Can you work these out from the model? Positions are in its coordinate system, mm. A direction names the side the tool comes from. Round coordinates to 2 decimals unless told otherwise and drop trailing zeros. Write each loop counter-clockwise with the first axis right and the second up, starting at its lowest first coordinate (ties: lowest second). Pieces come first, ordered by that corner, then holes. Notation, with made-up numbers: (87.5, -24) -> (135.5, -24) arc R27 ccw to (135.5, 10) -> close; hole circle Ø6 at (53, 23). An arc over 180 degrees is marked (long way). Write item = value, one per line. Start each with the question number.
1) Imagine slicing it at B-B, the plane y = -6.25. Please give me the cut outline in (x, z).
2) For faces 4 (the face through (-3.55, -11, 2)), 5 (the face through (-7, -1, -9)), 6 (the face through (-8, -11, -13.8)), which set-ups out of +Z, -Z, +X, -X, +Y, -Y let a thin tool reach every point of the face, with its end or its side?
3) If I drill on line 1 (Z direction, x = 0, y = -7); line 2 (Z direction, x = 7, y = -6); line 3 (Y direction, x = 0, z = 2.5), over which ranges is the centre line in solid material (lowest first)?
4) Imagine slicing it at C-C, the plane x = 6. Please give me the cut outline in (y, z), then the cut area to 3 significant figures.
5) Imagine slicing it at D-D, the plane z = 3.75. Please give me the cut outline in (x, y), then the cut area to 3 significant figures.
6) Thinking about a two-plate mould opening in Y: for faces 1 (the face through (-7.35, -4.8, -12.56)), 2 (the face through (8.91, 0.27, -0.07)), 3 (the face through (8.2, -13, -9.7)), which applies, +Y half, -Y half, draft (parallel to the pull), parting line (faces both ways), or undercut?
7) Imagine slicing it at A-A, the plane y = -2.5. Please give me the cut outline in (x, z).
8) I'm going to push flat-ended pins straight in: pin 1 (1.7 mm diameter, centred on x = 6, z = -11.5, fed in from +Y); pin 2 (5 mm diameter, centred on x = 7.5, z = -5, fed in from +Y); pin 3 (1.5 mm diameter, centred on x = -0.5, z = -7.5, fed in from +Y). Where does each tip first touch, or does it pass through?
from build123d import *

# Parameters (mm, degrees)
SKETCH1_R                       = 4
BOSS_EXTRUDE1_DEPTH             = 5
BOSS_EXTRUDE2_DEPTH             = 10
BOSS_EXTRUDE2_DIRECTION_2_REACH = 23.477
CUT_EXTRUDE1_REACH              = 33.229
CUT_EXTRUDE1_END_RADIUS         = 4
SKETCH2_R                       = 2.1
CUT_EXTRUDE2_START              = -3.5
CUT_EXTRUDE2_DEPTH              = 5.5
FILLET1_R                       = 5
SKETCH5_R                       = 1.6
CUT_EXTRUDE3_DEPTH              = 32.228992939
CUT_EXTRUDE4_START              = -4
CUT_EXTRUDE4_DEPTH              = 4.5


with BuildPart() as part:
    # Sketch1 → Boss-Extrude1 (new, symmetric)
    with BuildSketch(Plane.XY):
        with BuildLine():
            Line((-8, -2.872281323), (-8, -17))
            Line((-8, -17), (8, -17))
            Line((8, -17), (8, -2.872281323))
            ThreePointArc((8, -2.872281323), (0, 8.5), (-8, -2.872281323))
        make_face()
        Circle(SKETCH1_R, mode=Mode.SUBTRACT)
    extrude(amount=BOSS_EXTRUDE1_DEPTH, both=True)

    # Sketch4 → Boss-Extrude2 (add)
    with BuildSketch(Plane(origin=(0, 0, -5), x_dir=(-1, 0, 0), z_dir=(0, 0, -1))):
        with BuildLine():
            Line((-10, -1), (-4.387482194, -1))
            ThreePointArc((-4.387482194, -1), (0, -4.5), (4.387482194, -1))
            Line((4.387482194, -1), (10, -1))
            Line((10, -1), (10, -17))
            Line((10, -17), (-10, -17))
            Line((-10, -17), (-10, -1))
        make_face()
    extrude(amount=BOSS_EXTRUDE2_DEPTH)

    # Boss-Extrude2 direction 2: up to this face of the body (flat: up to its plane)
    boss_extrude2_direction_2_end = Plane(part.part.faces().sort_by_distance((0, -5.649299223, 5))[0])
    # Sketch4 → Boss-Extrude2 direction 2 (add, up to the picked face)
    with BuildSketch(Plane(origin=(0, 0, -5), x_dir=(-1, 0, 0), z_dir=(0, 0, -1)), mode=Mode.PRIVATE) as boss_extrude2_direction_2_sk1:
        with BuildLine():
            Line((-10, -1), (-4.387482194, -1))
            ThreePointArc((-4.387482194, -1), (0, -4.5), (4.387482194, -1))
            Line((4.387482194, -1), (10, -1))
            Line((10, -1), (10, -17))
            Line((10, -17), (-10, -17))
            Line((-10, -17), (-10, -1))
        make_face()
    boss_extrude2_direction_2_tool1 = split(extrude(boss_extrude2_direction_2_sk1.sketch, amount=-BOSS_EXTRUDE2_DIRECTION_2_REACH, mode=Mode.PRIVATE), bisect_by=boss_extrude2_direction_2_end, keep=Keep.BOTH, mode=Mode.PRIVATE)
    add(boss_extrude2_direction_2_tool1.solids().sort_by(Axis((0, -9.503652, -5), (0, 0, 1)))[0])

    # Cut-Extrude1: up to this cylinder (the profile starts outside it)
    cut_extrude1_end = Plane(origin=(0, 0, 0), z_dir=(0, 0, -1)) * Cylinder(CUT_EXTRUDE1_END_RADIUS, 75.458, mode=Mode.PRIVATE)
    # Sketch2 → Cut-Extrude1 (cut, up to the surface)
    with BuildSketch(Plane.XZ.offset(17), mode=Mode.PRIVATE) as cut_extrude1_sk1:
        with Locations(Location((0, 0, 0), (0, 0, 270))):
            Circle(SKETCH2_R)
    cut_extrude1_tool1 = extrude(cut_extrude1_sk1.sketch, amount=-CUT_EXTRUDE1_REACH, mode=Mode.PRIVATE) - cut_extrude1_end
    add(cut_extrude1_tool1.solids().sort_by_distance((0, -17, 0))[0], mode=Mode.SUBTRACT)

    # Sketch3 → Cut-Extrude2 (cut)
    with BuildSketch(Plane.XZ.offset(17).offset(CUT_EXTRUDE2_START)):
        Polygon((-3.55, 2.049593456), (-3.55, 5), (3.55, 5), (3.55, 2.049593456), (3.55, -2.049593456), (0, -4.099186911), (-3.55, -2.049593456), align=None)
    extrude(amount=-CUT_EXTRUDE2_DEPTH, mode=Mode.SUBTRACT)

    # Fillet1
    # the kernel refuses this fillet: 5 mm, written as the material it adds along each edge
    with BuildSketch(Plane(origin=(-8.440971508, -1, -5), x_dir=(-1, 0, 0), z_dir=(0, 0, 1))) as fillet1_piece_1:
        with BuildLine():
            CenterArc((4.755970452, -3.844419605), FILLET1_R, 129.746228544, 38.09052624)
            Line((-0.131785829, -2.790930863), (-0.229540955, -2.769861088))
            ThreePointArc((-0.229540955, -2.769861088), (-0.050320463, -1.396200752), (-0.099305547, -0.011764706))
            Line((-0.099305547, -0.011764706), (0, 0.1))
            ThreePointArc((0, 0.1), (0.779514246, 0.1), (1.495089653, 0.076888392))
            Line((1.495089653, 0.076888392), (1.559028492, 0))
        make_face()
    extrude(amount=10)
    with BuildSketch(Plane(origin=(8.440971508, -1, -5), x_dir=(1, 0, 0), z_dir=(0, 0, 1))) as fillet1_piece_2:
        with BuildLine():
            CenterArc((4.755970452, 3.844419605), FILLET1_R, 192.163245216, 38.09052624)
            Line((-0.131785829, 2.790930863), (-0.229540955, 2.769861088))
            ThreePointArc((-0.229540955, 2.769861088), (-0.050320463, 1.396200752), (-0.099305547, 0.011764706))
            Line((-0.099305547, 0.011764706), (0, -0.1))
            ThreePointArc((0, -0.1), (0.779514246, -0.1), (1.495089653, -0.076888392))
            Line((1.495089653, -0.076888392), (1.559028492, 0))
        make_face()
    extrude(amount=10)

    # Sketch5 → Cut-Extrude3 (cut, through all)
    with BuildSketch(Plane.XZ.offset(17)):
        with Locations((7, -11)):
            Circle(SKETCH5_R)
        with Locations((-7, -11)):
            Circle(SKETCH5_R)
    extrude(amount=-CUT_EXTRUDE3_DEPTH, mode=Mode.SUBTRACT)

    # Sketch6 → Cut-Extrude4 (cut)
    with BuildSketch(Plane.XZ.offset(17).offset(CUT_EXTRUDE4_START)):
        Polygon((-8.616580754, -8.2), (-10, -8.2), (-10, -13.8), (-8.616580754, -13.8), (-5.383419246, -13.8), (-3.766838493, -11), (-5.383419246, -8.2), align=None)
        Polygon((8.616580754, -8.2), (5.383419246, -8.2), (3.766838493, -11), (5.383419246, -13.8), (8.616580754, -13.8), (10, -13.8), (10, -8.2), align=None)
    extrude(amount=-CUT_EXTRUDE4_DEPTH, mode=Mode.SUBTRACT)


solid = part.part
Reported:
q1.outline = (-10, -15) -> (10, -15) -> (10, 5) -> (-10, 5) -> close; hole circle Ø3.2 at (-7, -11); hole circle Ø4.2 at (0, 0); hole circle Ø3.2 at (7, -11)
q2.face_4 = +Z
q2.face_5 = -Z, +X, -X, +Y
q2.face_6 = -X
q3.line_1 = -15 to -2.1, 2.1 to 5
q3.line_2 = -15 to -12.6, -9.4 to 5
q3.line_3 = -17 to -13.5, -8 to -4, 4 to 8.5
q4.outline = (-17, -15) -> (-1, -15) -> (-1, -12.25) -> (-8.5, -12.25) -> (-8.5, -13.8) -> (-13, -13.8) -> (-13, -12.25) -> (-17, -12.25) -> close; (-17, -9.75) -> (-13, -9.75) -> (-13, -8.2) -> (-8.5, -8.2) -> (-8.5, -9.75) -> (-1, -9.75) -> (-1, -5) -> (6.02, -5) -> (6.02, 5) -> (-17, 5) -> close
q4.area = 336 mm²
q5.outline = (-10, -17) -> (10, -17) -> (10, -1) arc R5 cw to (8.31, 1.79) arc R8.5 ccw to (-8.31, 1.79) arc R5 cw to (-10, -1) -> close; hole circle Ø8 at (0, 0); hole (-3.55, -13.5) -> (3.55, -13.5) -> (3.55, -8) -> (-3.55, -8) -> close
q5.area = 364 mm²
q6.face_1 = draft
q6.face_2 = +Y half
q6.face_3 = undercut
q7.outline = (-10, -15) -> (-3.74, -15) -> (-3.74, -5) -> (-3.12, -5) -> (-3.12, 5) -> (-10, 5) -> close; (3.12, -5) -> (3.74, -5) -> (3.74, -15) -> (10, -15) -> (10, 5) -> (3.12, 5) -> close; hole circle Ø3.2 at (-7, -11); hole circle Ø3.2 at (7, -11)
q8.pin_1 = -1
q8.pin_2 = 6.87
q8.pin_3 = -4.32
